The model under review builds one solid part; all positions refer to its coordinate system, in mm. A direction names the side the tool comes from. Coordinates: 2 decimals unless noted, no trailing zeros. Order: outer loops, then holes, each group sorted by start corner. A loop starts at its lowest first (then second) coordinate and runs counter-clockwise, first axis right, second up. Notation, with made-up numbers: (7.25, -25) -> (11.25, -25) arc R23 ccw to (11.25, -15) -> close; hole circle Ø5 at (-25, 75). An arc over 180 degrees is marked (long way). Put each result on its own line as item: value.
from build123d import *

# Parameters (mm, degrees)
SKETCH002_AS_DRAWN_W                      = 0.64
SKETCH002_AS_DRAWN_H                      = 0.64
EXTRUDE002_DEPTH                          = 6
EXTRUDE002_ONTO_SKETCH002_ROLL_ANGLE      = 90
CHAMFER001_SIZE                           = 0.15
SKETCH003_W                               = 0.8
SKETCH003_H                               = 1.9
EXTRUDE003_DEPTH                          = 7.62
EXTRUDE001_DEPTH                          = 2.5
EXTRUDE001_ONTO_SKETCH001_ROLL_ANGLE      = 90
SKETCH_AS_DRAWN_W                         = 7.62
SKETCH_AS_DRAWN_H                         = 2.5
EXTRUDE_DEPTH                             = 2.5
EXTRUDE_ONTO_SKETCH_ROLL_ANGLE            = 90
CHAMFER_SIZE                              = 0.3
SKETCH004_AS_DRAWN_W                      = 0.64
SKETCH004_AS_DRAWN_H                      = 1.57
EXTRUDE004_DEPTH                          = 3.8
EXTRUDE004_ONTO_SKETCH004_ROLL_ANGLE      = 90
EXTRUDE004_ONTO_SKETCH004_PLACEMENT_ANGLE = 180
EXTRUDE005_DEPTH                          = 5.72
FILLET_R                                  = 0.2
CHAMFER002_SIZE                           = 0.15


with BuildPart() as chamfer001:
    # Sketch002 as drawn → Extrude002 (new)
    with BuildSketch(Plane.XY):
        Rectangle(SKETCH002_AS_DRAWN_W, SKETCH002_AS_DRAWN_H)
        with Locations((-2.54, 0)):
            Rectangle(SKETCH002_AS_DRAWN_W, SKETCH002_AS_DRAWN_H)
        with Locations((2.54, 0)):
            Rectangle(SKETCH002_AS_DRAWN_W, SKETCH002_AS_DRAWN_H)
    extrude(amount=EXTRUDE002_DEPTH)


with BuildPart() as chamfer001_1:
    # Extrude002 onto Sketch002 roll: moved
    add(chamfer001.part.rotate(Axis((0, 0, 0), (1, 0, 0)), EXTRUDE002_ONTO_SKETCH002_ROLL_ANGLE))


with BuildPart() as chamfer001_2:
    # Extrude002 onto Sketch002 placement: moved
    add(chamfer001_1.part.moved(Location((0, -2.5, 0))))

    # Chamfer001
    chamfer001_edges = [chamfer001_2.edges().sort_by_distance(p)[0] for p in [
        (0, -8.5, 0.32),
        (-0.32, -8.5, 0),
        (0, -8.5, -0.32),
        (0.32, -8.5, 0),
        (2.54, -8.5, 0.32),
        (2.22, -8.5, 0),
        (2.54, -8.5, -0.32),
        (2.86, -8.5, 0),
        (-2.54, -8.5, 0.32),
        (-2.86, -8.5, 0),
        (-2.54, -8.5, -0.32),
        (-2.22, -8.5, 0),
    ]]
    chamfer(chamfer001_edges, length=CHAMFER001_SIZE)


with BuildPart() as extrude003:
    # Sketch003 (on Face6 of Cut) → Extrude003 (new body)
    with BuildSketch(Plane(origin=(-3.81, 0, 0), x_dir=(0, -1, 0), z_dir=(-1, 0, 0))):
        with Locations((0.4, 0)):
            Rectangle(SKETCH003_W, SKETCH003_H)
    extrude(amount=-EXTRUDE003_DEPTH)


with BuildPart() as extrude001:
    # Sketch001 as drawn → Extrude001 (new)
    with BuildSketch(Plane.XY):
        Polygon((-1.57, 1.25), (-1.27, 0.95), (-0.97, 1.25), align=None)
        Polygon((1.57, 1.25), (1.27, 0.95), (0.97, 1.25), align=None)
        Polygon((-1.57, -1.25), (-1.27, -0.95), (-0.97, -1.25), align=None)
        Polygon((1.57, -1.25), (1.27, -0.95), (0.97, -1.25), align=None)
    extrude(amount=-EXTRUDE001_DEPTH)


with BuildPart() as extrude001_1:
    # Extrude001 onto Sketch001 roll: moved
    add(extrude001.part.rotate(Axis((0, 0, 0), (1, 0, 0)), EXTRUDE001_ONTO_SKETCH001_ROLL_ANGLE))


with BuildPart() as extrude001_2:
    # Extrude001 onto Sketch001 placement: moved
    add(extrude001_1.part.moved(Location((0, -2.5, 0))))


with BuildPart() as cut001:
    # Sketch as drawn → Extrude (new)
    with BuildSketch(Plane.XY):
        Rectangle(SKETCH_AS_DRAWN_W, SKETCH_AS_DRAWN_H)
    extrude(amount=EXTRUDE_DEPTH)


with BuildPart() as cut001_1:
    # Extrude onto Sketch roll: moved
    add(cut001.part.rotate(Axis((0, 0, 0), (1, 0, 0)), EXTRUDE_ONTO_SKETCH_ROLL_ANGLE))


with BuildPart() as cut001_2:
    # Extrude onto Sketch placement: moved
    add(cut001_1.part)

    # Chamfer
    chamfer_edges = [cut001_2.edges().sort_by_distance(p)[0] for p in [
        (-3.81, -1.25, 1.25),
        (3.81, -1.25, 1.25),
        (3.81, -1.25, -1.25),
        (-3.81, -1.25, -1.25),
    ]]
    chamfer(chamfer_edges, length=CHAMFER_SIZE)

    # Cut: cut Extrude001
    add(extrude001_2.part, mode=Mode.SUBTRACT)

    # Cut001: cut Extrude003
    add(extrude003.part, mode=Mode.SUBTRACT)


with BuildPart() as extrude004:
    # Sketch004 as drawn → Extrude004 (new)
    with BuildSketch(Plane.XY):
        with Locations((0, -0.465)):
            Rectangle(SKETCH004_AS_DRAWN_W, SKETCH004_AS_DRAWN_H)
        with Locations((-2.54, -0.465)):
            Rectangle(SKETCH004_AS_DRAWN_W, SKETCH004_AS_DRAWN_H)
        with Locations((2.54, -0.465)):
            Rectangle(SKETCH004_AS_DRAWN_W, SKETCH004_AS_DRAWN_H)
    extrude(amount=EXTRUDE004_DEPTH)


with BuildPart() as extrude004_1:
    # Extrude004 onto Sketch004 roll: moved
    add(extrude004.part.rotate(Axis((0, 0, 0), (1, 0, 0)), EXTRUDE004_ONTO_SKETCH004_ROLL_ANGLE))


with BuildPart() as extrude004_2:
    # Extrude004 onto Sketch004 placement: moved
    add(extrude004_1.part.moved(Location((0, -0.8, 0))).rotate(Axis((0, -0.8, 0), (0, 0, 1)), EXTRUDE004_ONTO_SKETCH004_PLACEMENT_ANGLE))


with BuildPart() as fusion:
    # Sketch005 (on Face8 of Extrude004) → Extrude005 (new body)
    with BuildSketch(Plane(origin=(-2.86, 0, 0), x_dir=(0, -1, 0), z_dir=(-1, 0, 0))):
        Polygon((0.8, 0.32), (0, 0.32), (-1.73, -0.61), (-3, -0.61), (-3, -1.25), (-1.73, -1.25), (0, -0.32), (0.8, -0.32), align=None)
    extrude(amount=-EXTRUDE005_DEPTH)

    # Common: intersect Extrude004
    add(extrude004_2.part, mode=Mode.INTERSECT)

    # Fillet
    fillet_edges = [fusion.edges().sort_by_distance(p)[0] for p in [
        (2.54, 1.73, -0.61),
        (2.54, 0, 0.32),
        (2.54, 0, -0.32),
        (2.54, 1.73, -1.25),
        (0, 1.73, -0.61),
        (0, 0, 0.32),
        (0, 0, -0.32),
        (0, 1.73, -1.25),
        (-2.54, 1.73, -0.61),
        (-2.54, 0, 0.32),
        (-2.54, 0, -0.32),
        (-2.54, 1.73, -1.25),
    ]]
    fillet(fillet_edges, radius=FILLET_R)

    # Chamfer002
    chamfer002_edges = [fusion.edges().sort_by_distance(p)[0] for p in [
        (2.54, 3, -0.61),
        (2.86, 3, -0.93),
        (2.22, 3, -0.93),
        (2.54, 3, -1.25),
        (0, 3, -0.61),
        (0.32, 3, -0.93),
        (-0.32, 3, -0.93),
        (0, 3, -1.25),
        (-2.54, 3, -0.61),
        (-2.22, 3, -0.93),
        (-2.86, 3, -0.93),
        (-2.54, 3, -1.25),
    ]]
    chamfer(chamfer002_edges, length=CHAMFER002_SIZE)

    # Fusion: union Chamfer001, Cut001
    add(chamfer001_2.part)
    add(cut001_2.part)


solid = fusion.part
Item 1: Consider section C-C on x = -2.5. Write out the cut boundary in (y, z), and give its area (3 significant figures).
Answers below:
outline: (-8.5, -0.17) -> (-8.35, -0.32) -> (-2.5, -0.32) -> (-2.5, -1.25) -> (0, -1.25) -> (0, -0.95) -> (-0.8, -0.95) -> (-0.8, -0.32) -> (-0.05, -0.32) arc R0.2 cw to (0.04, -0.34) -> (1.69, -1.23) arc R0.2 ccw to (1.78, -1.25) -> (2.85, -1.25) -> (3, -1.1) -> (3, -0.76) -> (2.85, -0.61) -> (1.78, -0.61) arc R0.2 cw to (1.69, -0.59) -> (0.04, 0.3) arc R0.2 ccw to (-0.05, 0.32) -> (-0.8, 0.32) -> (-0.8, 0.95) -> (0, 0.95) -> (0, 1.25) -> (-2.5, 1.25) -> (-2.5, 0.32) -> (-8.35, 0.32) -> (-8.5, 0.17) -> close
area: 11.0 mm^2
Item 2: Consider section D-D on z = 0.5. Write out the cut boundary in (x, y), and give its area (3 significant figures).
Answers below:
outline: (-3.81, -2.5) -> (3.81, -2.5) -> (3.81, -0.8) -> (-3.81, -0.8) -> close
area: 13.0 mm^2
Item 3: Consider section A-A on y = -4.75. Write out the cut boundary in (x, z).
Answers below:
outline: (-2.86, -0.32) -> (-2.22, -0.32) -> (-2.22, 0.32) -> (-2.86, 0.32) -> close; (-0.32, -0.32) -> (0.32, -0.32) -> (0.32, 0.32) -> (-0.32, 0.32) -> close; (2.22, -0.32) -> (2.86, -0.32) -> (2.86, 0.32) -> (2.22, 0.32) -> close
Item 4: For line 1 (Z direction, x = 2.5, y = -0.5); line 2 (Z direction, x = 0, y = -5), list the stretches that pass through material, from the lowest coordinate up. Write a range as from..to.
Answers below:
line 1: -1.25..-0.95, -0.32..0.32, 0.95..1.25
line 2: -0.32..0.32
Item 5: Consider section B-B on y = -1.25. Write out the cut boundary in (x, z).
Answers below:
outline: (-3.81, -0.95) -> (-3.51, -1.25) -> (-1.57, -1.25) -> (-1.27, -0.95) -> (-0.97, -1.25) -> (0.97, -1.25) -> (1.27, -0.95) -> (1.57, -1.25) -> (3.51, -1.25) -> (3.81, -0.95) -> (3.81, 0.95) -> (3.51, 1.25) -> (1.57, 1.25) -> (1.27, 0.95) -> (0.97, 1.25) -> (-0.97, 1.25) -> (-1.27, 0.95) -> (-1.57, 1.25) -> (-3.51, 1.25) -> (-3.81, 0.95) -> close
Item 6: Mouldability with a two-part tool opening along Y and no side actions: class faces 6 (the flat face through (-2.544, 0.854, -0.139)), 7 (the flat face through (-3.81, -2, 0)), 8 (the flat face through (-0.004, 0.876, -0.791)), 9 (the flat face through (2.536, 0.876, -0.791)) as +Y half, -Y half, draft (parallel to the pull), parting line (faces both ways), or undercut.
Answers below:
face 6: +Y half
face 7: draft
face 8: undercut
face 9: undercut
Item 7: For pin 1 Ø0.7 at (y, z) = (-5, 0) entering from -X; pin 2 Ø0.7 at (y, z) = (-5, 0) entering from +X; pin 3 Ø3 at (x, y) = (3, -6.5) entering from +Z, all flat-tipped, find the tip position at first contact; note any pin that passes through.
Answers below:
pin 1: x = -2.86
pin 2: x = 2.86
pin 3: z = 0.32
Item 8: For faces 1 (the flat face through (2.86, 1.1, -0.5)), 2 (the flat face through (2.5, -0.4, 0.95)), 3 (the flat face through (-2.544, 0.876, -0.791)), 4 (the flat face through (-0.1, -0.8, -0.6)), 5 (the flat face through (-0.32, 1, -0.5)), list the 3-axis set-ups (+Z, -Z, +X, -X, +Y, -Y) from which the entire face can be reached by the end or side of a thin tool; tool diameter is ignored.
Answers below:
face 1: +X, +Y
face 2: +X, -X, +Y
face 3: -Z, +X, -X
face 4: none
face 5: +Y
